For this review, take the finished solid that the model builds, in its own axes (mm). A direction names the side the tool comes from. Coordinates: 2 decimals unless noted, no trailing zeros. Write each loop counter-clockwise with the first axis right and the second up, starting at its lowest first coordinate (ties: lowest second). Pieces come first, ordered by that corner, then holes.
Autodesk Inventor part; units mm, degrees
ref_plane "side_4d_XY" through (-20, 0, -330) normal (-1, 0, 0) x (0, 1, 0)
ref_plane "side_4d_YZ" through (-20, 0, -330) normal (0, 1, 0) x (0, 0, -1)
ref_plane "side_4d_ZX" through (-20, 0, -330) normal (0, 0, -1) x (-1, 0, 0)
sketch "Skizze_1" plane through (0, 0, 0) normal (0, 0, 1) x (1, 0, 0)
  arc A0 (-20, -17) -> (-17, -20) centre (-17, -17) ccw
  line L0 (-17, -20) -> (-4.1, -20)
  line L1 (-4.1, -20) -> (-4.1, -17)
  line L2 (-4.1, -17) -> (-10.5, -17)
  line L3 (-10.5, -17) -> (-10.5, -13.6627)
  arc A1 (-10.0314, -12.5314) -> (-10.5, -13.6627) centre (-8.9002, -13.6627) ccw
  line L4 (-10.0314, -12.5314) -> (-7.4645, -9.9645)
  arc A2 (-3.9289, -8.5) -> (-7.4645, -9.9645) centre (-3.9289, -13.5) ccw
  line L5 (-3.9289, -8.5) -> (3.9289, -8.5)
  arc A3 (7.4645, -9.9645) -> (3.9289, -8.5) centre (3.9289, -13.5) ccw
  line L6 (7.4645, -9.9645) -> (10.0314, -12.5314)
  arc A4 (10.5, -13.6627) -> (10.0314, -12.5314) centre (8.9002, -13.6627) ccw
  line L7 (10.5, -13.6627) -> (10.5, -17)
  line L8 (10.5, -17) -> (4.1, -17)
  line L9 (4.1, -17) -> (4.1, -20)
  line L10 (4.1, -20) -> (17, -20)
  arc A5 (17, -20) -> (20, -17) centre (17, -17) ccw
  line L11 (20, -17) -> (20, -4.1)
  line L12 (20, -4.1) -> (17, -4.1)
  line L13 (17, -4.1) -> (17, -10.5)
  line L14 (17, -10.5) -> (13.6627, -10.5)
  arc A6 (12.5314, -10.0314) -> (13.6627, -10.5) centre (13.6627, -8.9002) ccw
  line L15 (12.5314, -10.0314) -> (9.9645, -7.4645)
  arc A7 (8.5, -3.9289) -> (9.9645, -7.4645) centre (13.5, -3.9289) ccw
  line L16 (8.5, -3.9289) -> (8.5, 3.9289)
  arc A8 (9.9645, 7.4645) -> (8.5, 3.9289) centre (13.5, 3.9289) ccw
  line L17 (9.9645, 7.4645) -> (12.5314, 10.0314)
  arc A9 (13.6627, 10.5) -> (12.5314, 10.0314) centre (13.6627, 8.9002) ccw
  line L18 (13.6627, 10.5) -> (17, 10.5)
  line L19 (17, 10.5) -> (17, 4.1)
  line L20 (17, 4.1) -> (20, 4.1)
  line L21 (20, 4.1) -> (20, 17)
  arc A10 (20, 17) -> (17, 20) centre (17, 17) ccw
  line L22 (17, 20) -> (4.1, 20)
  line L23 (4.1, 20) -> (4.1, 17)
  line L24 (4.1, 17) -> (10.5, 17)
  line L25 (10.5, 17) -> (10.5, 13.6627)
  arc A11 (10.0314, 12.5314) -> (10.5, 13.6627) centre (8.9002, 13.6627) ccw
  line L26 (10.0314, 12.5314) -> (7.4645, 9.9645)
  arc A12 (3.9289, 8.5) -> (7.4645, 9.9645) centre (3.9289, 13.5) ccw
  line L27 (3.9289, 8.5) -> (-3.9289, 8.5)
  arc A13 (-7.4645, 9.9645) -> (-3.9289, 8.5) centre (-3.9289, 13.5) ccw
  line L28 (-7.4645, 9.9645) -> (-10.0314, 12.5314)
  arc A14 (-10.5, 13.6627) -> (-10.0314, 12.5314) centre (-8.9002, 13.6627) ccw
  line L29 (-10.5, 13.6627) -> (-10.5, 17)
  line L30 (-10.5, 17) -> (-4.1, 17)
  line L31 (-4.1, 17) -> (-4.1, 20)
  line L32 (-4.1, 20) -> (-17, 20)
  arc A15 (-17, 20) -> (-20, 17) centre (-17, 17) ccw
  line L33 (-20, 17) -> (-20, 4.1)
  line L34 (-20, 4.1) -> (-17, 4.1)
  line L35 (-17, 4.1) -> (-17, 10.5)
  line L36 (-17, 10.5) -> (-13.6627, 10.5)
  arc A16 (-12.5314, 10.0314) -> (-13.6627, 10.5) centre (-13.6627, 8.9002) ccw
  line L37 (-12.5314, 10.0314) -> (-9.9645, 7.4645)
  arc A17 (-8.5, 3.9289) -> (-9.9645, 7.4645) centre (-13.5, 3.9289) ccw
  line L38 (-8.5, 3.9289) -> (-8.5, -3.9289)
  arc A18 (-9.9645, -7.4645) -> (-8.5, -3.9289) centre (-13.5, -3.9289) ccw
  line L39 (-9.9645, -7.4645) -> (-12.5314, -10.0314)
  arc A19 (-13.6627, -10.5) -> (-12.5314, -10.0314) centre (-13.6627, -8.9002) ccw
  line L40 (-13.6627, -10.5) -> (-17, -10.5)
  line L41 (-17, -10.5) -> (-17, -4.1)
  line L42 (-17, -4.1) -> (-20, -4.1)
  line L43 (-20, -4.1) -> (-20, -17)
  circle A20 centre (0, 0) radius 6
extrude "Extrusion1" add sketch "Skizze_1" against normal blind 100
sketch "Sketch2" plane through (0, 0, 0) normal (0, 0, 1) x (1, 0, 0)
  point P0 (-15, -15)
hole "Drilling 1" at (-15, -15, 0) direction (0, 0, -1) diameter 5 depth 6000
sketch "Sketch3" plane through (0, 0, 0) normal (0, 0, 1) x (1, 0, 0)
  point P0 (15, -15)
hole "Drilling 2" at (15, -15, 0) direction (0, 0, -1) diameter 5 depth 6000
sketch "Sketch4" plane through (0, 0, 0) normal (0, 0, 1) x (1, 0, 0)
  point P0 (15, 15)
hole "Drilling 3" at (15, 15, 0) direction (0, 0, -1) diameter 5 depth 6000
sketch "Sketch5" plane through (0, 0, 0) normal (0, 0, 1) x (1, 0, 0)
  point P0 (-15, 15)
hole "Drilling 4" at (-15, 15, 0) direction (0, 0, -1) diameter 5 depth 6000
ref_plane "side_4d_XY" through (-20, 0, -330) normal (-1, 0, 0) x (0, 1, 0)
ref_plane "side_4d_YZ" through (-20, 0, -330) normal (0, 1, 0) x (0, 0, -1)
ref_plane "side_4d_ZX" through (-20, 0, -330) normal (0, 0, -1) x (-1, 0, 0)
ref_plane "side_1a_XY" through (0, 20, -330) normal (0, 1, 0) x (1, 0, 0)
ref_plane "side_1a_YZ" through (0, 20, -330) normal (1, 0, 0) x (0, 0, -1)
ref_plane "side_1a_ZX" through (0, 20, -330) normal (0, 0, -1) x (0, 1, 0)
ref_plane "side_2b_XY" through (20, 0, -330) normal (1, 0, 0) x (0, -1, 0)
ref_plane "side_2b_YZ" through (20, 0, -330) normal (0, -1, 0) x (0, 0, -1)
ref_plane "side_2b_ZX" through (20, 0, -330) normal (0, 0, -1) x (1, 0, 0)
ref_plane "side_3c_XY" through (0, -20, -330) normal (0, -1, 0) x (-1, 0, 0)
ref_plane "side_3c_YZ" through (0, -20, -330) normal (-1, 0, 0) x (0, 0, -1)
ref_plane "side_3c_ZX" through (0, -20, -330) normal (0, 0, -1) x (0, -1, 0)
ref_plane "end_XY" through (0, 0, -660) normal (0, 0, -1) x (1, 0, 0)
ref_plane "end_YZ" through (0, 0, -660) normal (1, 0, 0) x (0, -1, 0)
ref_plane "end_ZX" through (0, 0, -660) normal (0, -1, 0) x (0, 0, -1)
ref_plane "start_XY" through (0, 0, 0) normal (0, 0, 1) x (1, 0, 0)
ref_plane "start_YZ" through (0, 0, 0) normal (1, 0, 0) x (0, 1, 0)
ref_plane "start_ZX" through (0, 0, 0) normal (0, 1, 0) x (0, 0, 1)
properties part number "MayTec 1.11.040040.43S_Profile 40x40, 4E, S_100_Detail_(0;0,0,0)"
Q1. Add section B-B (y = 0). State the section outline as (x, z) points.
Ans:
outline: (-8.5, -100) - (-6, -100) - (-6, 0) - (-8.5, 0) - close; (6, -100) - (8.5, -100) - (8.5, 0) - (6, 0) - close
Q2. For probe 1 along Y at (x, z) = (-15, -51); probe 2 along Y at (x, z) = (-7, -89), list the stretches that pass through material, from the lowest coordinate up.
Ans:
probe 1: y = -20 to -17.5, -12.5 to -10.5, 10.5 to 12.5, 17.5 to 20
probe 2: y = -20 to -17, -9.55 to 9.55, 17 to 20
Q3. Add section A-A (x = -15). State the section outline as (y, z) points.
Ans:
outline: (-20, -100) - (-17.5, -100) - (-17.5, 0) - (-20, 0) - close; (-12.5, -100) - (-10.5, -100) - (-10.5, 0) - (-12.5, 0) - close; (10.5, -100) - (12.5, -100) - (12.5, 0) - (10.5, 0) - close; (17.5, -100) - (20, -100) - (20, 0) - (17.5, 0) - close
Q4. Clearance check with flat-ended pins moving along their axes: pin 1 Ø0.9 at (x, z) = (-18.5, -64.5) entering from -Y; pin 2 Ø0.9 at (x, z) = (18, -52) entering from +Y; pin 3 Ø2.5 at (x, z) = (-1, -40) entering from -Y. State where each tip first meets the part, or that it passes through.
Ans:
pin 1: stops at y = -19.81
pin 2: stops at y = 19.95
pin 3: stops at y = -8.5
Q5. Add section D-D (z = -30.5). Give the number of separate pieces and of enclosed holes in the cut face, then the cut area to 3 significant figures.
Ans:
separate pieces: 1
enclosed holes: 5
area: 674 mm2
Q6. Draft analysis for pull direction Y (two halves, no side actions). For faces 1 (the flat face through (-19, 4.1, -49)), 2 (the flat face through (10, -20, -49)), 3 (the flat face through (-5, -4, 0)), state which applies: +Y half, -Y half, draft (parallel to the pull), parting line (faces both ways), or undercut.
Ans:
face 1: undercut
face 2: -Y half
face 3: draft
Q7. Tool access review of faces 4 (the flat face through (-18, -4.1, -49)), 5 (the flat face through (18, 4.1, -49)), 6 (the cylindrical face through (8.87, -5.82, -49.3)): name each direction out of +Z, -Z, +X, -X, +Y, -Y from which nothing blocks a thin tool from reaching the whole face with its end or side.
Ans:
face 4: +Z, -Z, -X
face 5: +Z, -Z, +X
face 6: +Z, -Z
